from build123d import *

# Parameters (mm, degrees)
SKETCH1_R           = 14
SKETCH1_W           = 14.5
SKETCH1_H           = 17
BOSS_EXTRUDE1_DEPTH = 19
SKETCH2_R           = 4.5
BOSS_EXTRUDE2_DEPTH = 1.5
SKETCH2_3_R         = 2.5
BOSS_EXTRUDE3_DEPTH = 10
CUT_EXTRUDE1_DEPTH  = 6
FILLET1_R           = 1
SKETCH4_R           = 2.1
BOSS_EXTRUDE4_DEPTH = 0.8


with BuildPart() as part:
    # Sketch1 → Boss-Extrude1 (new body)
    with BuildSketch(Plane(origin=(0, 0, 0), x_dir=(1, 0, 0), z_dir=(0, 1, 0))):
        Circle(SKETCH1_R)
        with Locations((0, -8.5)):
            Rectangle(SKETCH1_W, SKETCH1_H)
    extrude(amount=BOSS_EXTRUDE1_DEPTH)

    # Sketch2 → Boss-Extrude2 (add)
    with BuildSketch(Plane(origin=(0, 19, 0), x_dir=(1, 0, 0), z_dir=(0, 1, 0))):
        with Locations((0, 8.000000036)):
            Circle(SKETCH2_R)
    extrude(amount=BOSS_EXTRUDE2_DEPTH)

    # Sketch2_3 → Boss-Extrude3 (add)
    with BuildSketch(Plane(origin=(0, 19, 0), x_dir=(1, 0, 0), z_dir=(0, 1, 0))):
        with Locations((0, 8.000000036)):
            Circle(SKETCH2_3_R)
    extrude(amount=BOSS_EXTRUDE3_DEPTH)

    # Sketch3 → Cut-Extrude1 (cut)
    with BuildSketch(Plane(origin=(0, 29, 0), x_dir=(1, 0, 0), z_dir=(0, 1, 0))):
        with BuildLine():
            Line((-1.5, 6.000000036), (-1.5, 10.000000036))
            ThreePointArc((-1.5, 10.000000036), (-2.5, 8.000000036), (-1.5, 6.000000036))
        make_face()
        with BuildLine():
            ThreePointArc((2.5, 8.000000036), (2.236067977, 9.118034025), (1.5, 10.000000036))
            Line((1.5, 10.000000036), (1.5, 6.000000036))
            ThreePointArc((1.5, 6.000000036), (2.236067977, 6.881966047), (2.5, 8.000000036))
        make_face()
    extrude(amount=-CUT_EXTRUDE1_DEPTH, mode=Mode.SUBTRACT)

    # Fillet1
    fillet1_edges = [part.edges().sort_by_distance(p)[0] for p in [
        (-7.25, 9.5, 17),
        (7.25, 9.5, 17),
        (7.25, 0, 14.488269784),
        (0, 0, -14),
        (0, 0, 17),
        (-7.25, 0, 14.488269784),
        (7.25, 9.5, 11.976539567),
        (-7.25, 9.5, 11.976539567),
    ]]
    fillet(fillet1_edges, radius=FILLET1_R)

    # Sketch4 → Boss-Extrude4 (add)
    with BuildSketch(Plane(origin=(0, 19, 0), x_dir=(1, 0, 0), z_dir=(0, 1, 0))):
        with BuildLine():
            Line((-17.502332169, 3.500000036), (17.497667831, 3.500000036))
            ThreePointArc((17.497667831, 3.500000036), (20.997667831, 3.6e-08), (17.497667831, -3.499999964))
            Line((17.497667831, -3.499999964), (-17.502332169, -3.499999964))
            ThreePointArc((-17.502332169, -3.499999964), (-21.002332169, 3.6e-08), (-17.502332169, 3.500000036))
        make_face()
        with Locations((17.497667831, 3.6e-08)):
            Circle(SKETCH4_R, mode=Mode.SUBTRACT)
        with Locations((-17.502332169, 3.6e-08)):
            Circle(SKETCH4_R, mode=Mode.SUBTRACT)
    extrude(amount=-BOSS_EXTRUDE4_DEPTH)


solid = part.part
Model file for the job. Use its own axes, mm. A direction names the side the tool comes from. Coordinates: 2 decimals unless noted, no trailing zeros. Loops run counter-clockwise (first coordinate to the right, second up) from the corner with the lowest first, then second, coordinate; pieces in that order, holes last. Notation, with made-up numbers: (-7.75, 41.25) -> (6.25, 41.25) arc R18 ccw to (6.25, 72.25) -> close; hole circle Ø9 at (51, 65.25). An arc over 180 degrees is marked (long way). Use one line per item in the form item = value. Start each with the question number.
(1) Cut at B-B on x = 0. Give the cut face in (y, z).
(2) Tool access for faces 1 (the cylindrical face through (-0.59, 19.74, -12.46)), 2 (the cylindrical face through (6.965, 0.301, 14.239)), 3 (the cylindrical face through (-6.965, 0.301, 14.239)): list every direction of +Z, -Z, +X, -X, +Y, -Y with a clear straight run to the whole face (end or side of a thin tool).
(3) Flat gauge pins, fed straight in: pin 1 (5 mm diameter, centred on x = 15, z = 0.5, fed in from +Y); pin 2 (4 mm diameter, centred on y = 25, z = -4.5, fed in from -X); pin 3 (12 mm diameter, centred on y = 9, z = -9, fed in from +X). Where does each tip first touch, or does it go through?
(4) Probe probe 1 along X at (y, z) = (18.4, 0); probe 2 along X at (y, z) = (11.5, 13); probe 3 along X at (y, z) = (17.5, 3.5). List the from-to ranges inside material, lowest first. Write a range as from..to.
(5) Cut at D-D on y = 24.25. Give the cut face in (x, z).
(6) Cut at A-A on z = 0. Give the cut face in (x, y), and give its area (3 significant figures).
(7) Cut at C-C on y = 14. Give the cut face in (x, z).
(8) Pull direction Z, two halves, no side cores. Call faces 4 (the cylindrical face through (-19.6, 18.6, -0.1)), 5 (the flat face through (1.5, 26, -8)), 6 (the cylindrical face through (-21, 18.6, 0.1)): pulls with the +Z half, pulls with the -Z half, needs draft (parallel to the pull), parting line crosses it, or undercut.
Values:
q1.outline = (0, -13) arc R1 ccw to (1, -14) -> (19, -14) -> (19, -12.5) -> (20.5, -12.5) -> (20.5, -10.5) -> (29, -10.5) -> (29, -5.5) -> (20.5, -5.5) -> (20.5, -3.5) -> (19, -3.5) -> (19, 17) -> (1, 17) arc R1 ccw to (0, 16) -> close
q2.face_1 = +Y
q2.face_2 = +Z, +X, -Y
q2.face_3 = +Z, -X, -Y
q3.pin_1 = 19
q3.pin_2 = -1.5
q3.pin_3 = 13.67
q4.probe_1 = -21..-19.6, -15.4..15.4, 19.6..21
q4.probe_2 = -7.25..7.25
q4.probe_3 = -13.56..13.56
q5.outline = (-1.5, -10) arc R2.5 ccw to (1.5, -10) -> (1.5, -6) arc R2.5 ccw to (-1.5, -6) -> close
q6.outline = (-21, 18.2) -> (-19.6, 18.2) -> (-19.6, 19) -> (-21, 19) -> close; (-15.4, 18.2) -> (-14, 18.2) -> (-14, 1) arc R1 ccw to (-13, 0) -> (13, 0) arc R1 ccw to (14, 1) -> (14, 18.2) -> (15.4, 18.2) -> (15.4, 19) -> (-15.4, 19) -> close; (19.6, 18.2) -> (21, 18.2) -> (21, 19) -> (19.6, 19) -> close
q6.area = 536 mm2
q7.outline = (-7.7, 11.69) arc R14 ccw (long way) to (7.7, 11.69) arc R1 cw to (7.25, 12.53) -> (7.25, 16) arc R1 ccw to (6.25, 17) -> (-6.25, 17) arc R1 ccw to (-7.25, 16) -> (-7.25, 12.53) arc R1 cw to start
q8.face_4 = undercut
q8.face_5 = needs draft
q8.face_6 = parting line crosses it
